Drawing for the job (mm, zero at the part's lowest x, y, z). A direction names the side the tool comes from. Round coordinates to 2 decimals unless told otherwise and drop trailing zeros. Order: outer loops, then holes, each group sorted by start corner. A loop starts at its lowest first (then second) coordinate and runs counter-clockwise, first axis right, second up. Notation, with made-up numbers: (8.5, 14.5) - (40.5, 14.5) arc R23 cw to (40.5, 46.5) - close; hole circle Ø8 at (87.25, -29.75). An arc over 180 degrees is marked (long way). Put each result on its own line as item: value. Start each with the question number.
Item 1: Pin check, flat tips, straight feed: pin 1 Ø5 at (y, z) = (42.5, 11.5) entering from +X; pin 2 Ø3 at (x, y) = (11, 44) entering from +Z; pin 3 Ø5 at (x, z) = (4, 29.5) entering from +Y. Stop position of each tip, or through.
Item 2: Saw through at C-C on x = 13.75. List the corners of the cut face in (y, z), plus the area to 3 significant figures.
Item 3: Saw through at D-D on y = 4. List the corners of the cut face in (x, z), plus the area to 3 significant figures.
Item 4: Which spindle directions (+Z, -Z, +X, -X, +Y, -Y) get a long thin tool onto all of the face, cutting with end or side? Do the marked faces 1 and 2. Say none if no direction does.
Item 5: Probe probe 1 along Y at (x, z) = (7, 49.5); probe 2 along Y at (x, z) = (4.5, 37). List the from-to ranges inside material, lowest first.
Item 6: Saw through at B-B on z = 13. List the corners of the cut face in (x, y).
Item 7: Saw through at A-A on y = 14. List the corners of the cut face in (x, z), plus the area to 3 significant figures.
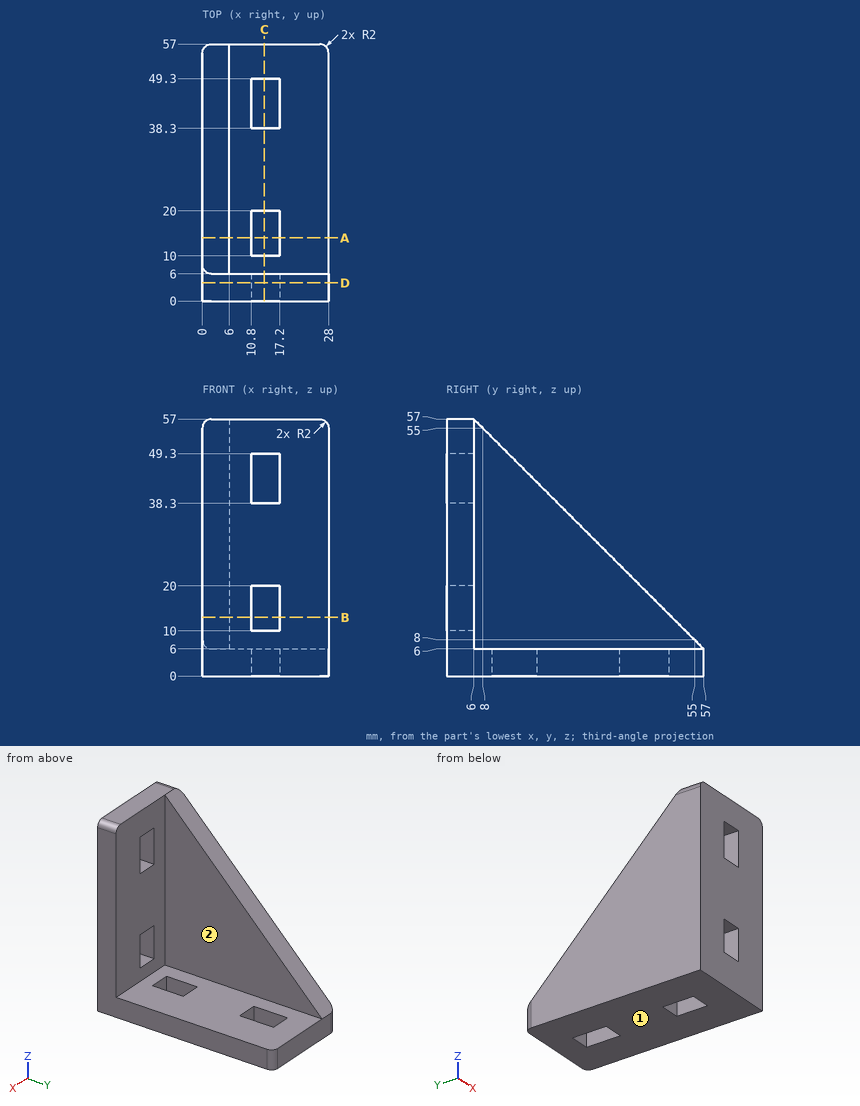
Results found:
1. pin 1: stops at x = 6
1. pin 2: stops at z = 6
1. pin 3: stops at y = 36
2. outline: (0, 0) - (10, 0) - (10, 6) - (6, 6) - (6, 10) - (0, 10) - close; (0, 20) - (6, 20) - (6, 38.3) - (0, 38.3) - close; (0, 49.3) - (6, 49.3) - (6, 57) - (0, 57) - close; (20, 0) - (38.3, 0) - (38.3, 6) - (20, 6) - close; (49.3, 0) - (57, 0) - (57, 6) - (49.3, 6) - close
2. area: 396 mm²
3. outline: (0, 0) - (28, 0) - (28, 55) arc R2 ccw to (26, 57) - (2, 57) arc R2 ccw to (0, 55) - close; hole (10.8, 10) - (17.2, 10) - (17.2, 20) - (10.8, 20) - close; hole (10.8, 38.3) - (17.2, 38.3) - (17.2, 49.3) - (10.8, 49.3) - close
3. area: 1,460 mm²
4. face 1: -Z, +X, -X, +Y, -Y
4. face 2: +Z, +X, +Y
5. probe 1: y = 0 to 6
5. probe 2: y = 0 to 26
6. outline: (0, 0) - (10.8, 0) - (10.8, 6) - (6, 6) - (6, 50) - (0, 50) - close; (17.2, 0) - (28, 0) - (28, 6) - (17.2, 6) - close
7. outline: (0, 0) - (10.8, 0) - (10.8, 6) - (6, 6) - (6, 49) - (0, 49) - close; (17.2, 0) - (28, 0) - (28, 6) - (17.2, 6) - close
7. area: 388 mm²
